Work out the finished part from the listing and answer in its coordinate system (mm). A direction names the side the tool comes from. Round coordinates to 2 decimals unless told otherwise and drop trailing zeros. Loops run counter-clockwise (first coordinate to the right, second up) from the corner with the lowest first, then second, coordinate; pieces in that order, holes last. Notation, with made-up numbers: (64, -17) - (108, -17) arc R16 ccw to (108, -13) - close; hole circle Ø5 at (81, -19). An arc over 180 degrees is marked (long way). Answer as CSV lines item,"result". Start each with the question number.
Q1. The mould has two halves that part along Z. Classify faces 4 (the face through (25, -2, -8.365)), 5 (the face through (37, -2, 12.675)), 6 (the face through (-6.727, 4.465, 32.917)), 7 (the face through (-9, 7, -5)): +Z half, -Z half, draft (parallel to the pull), parting line (faces both ways), or undercut.
Q2. Section B-B on y = 2.75 is taken. Write down the section's boundary in (x, z).
Q3. Section C-C on y = -1 is taken. Write down the section's boundary in (x, z).
Q4. Section A-A on x = 37 is taken. Write down the section's boundary in (y, z), then the cut area to 3 significant figures.
Q5. Each of these flat-tipped pins is pushed along its axis until it touches: pin 1 Ø1 at (y, z) = (3.5, -1.5) entering from -X; pin 2 Ø6 at (y, z) = (4.5, 0) entering from +X; pin 3 Ø3.5 at (x, z) = (-6.64, 34.92) entering from +Y. Where does it stop, or does it pass through?
Q6. Section D-D on z = 10.5 is taken. Write down the section's boundary in (x, y).
Q7. For faces 1 (the face through (15.52, -2.22, 15.33)), 2 (the face through (53.99, 4.46, 33.44)), 3 (the face through (24, -4.5, 16)), determine the directions among +Z, -Z, +X, -X, +Y, -Y from which every point of the face is accessible in a straight line to the end or side of a thin tool.
Q8. Straight lines are drawn through the part: L1, parallel to X at y = -2, z = 13.5; L2, parallel to Y at x = 21, z = 31; L3, parallel to X at y = -3.5, z = -4.5. For each, find the intervals that lie inside material, in ascending order. Write a range as [from, to].
Autodesk Inventor part; units mm, degrees
ref_plane "YZ Plane" through (0, 0, 0) normal (1, 0, 0) x (0, 1, 0)
ref_plane "XZ Plane" through (0, 0, 0) normal (0, 1, 0) x (-1, 0, 0)
ref_plane "XY Plane" through (0, 0, 0) normal (0, 0, 1) x (1, 0, 0)
sketch "proto-board hole layout" plane through (0, 0, 0) normal (0, 1, 0) x (-1, 0, 0)
  circle A0 centre (6.6395, -4.3647) radius 1.49
  circle A1 centre (-55.3405, -4.3647) radius 1.49
  circle A2 centre (-55.3405, 34.9153) radius 1.49
  circle A3 centre (6.6395, 34.9153) radius 1.49
  line L0 (5.1495, -4.3647) -> (-53.8505, -4.3647) construction
  line L1 (5.1495, 34.9153) -> (-53.8505, 34.9153) construction
  line L2 (-55.3405, 33.4253) -> (-55.3405, -2.8747) construction
  line L3 (6.6395, 33.4253) -> (6.6395, -2.8747) construction
  dimension "d0" = 2.98
  dimension "d1" = 59
  dimension "d2" = 36.3
sketch "Sketch3" plane through (0, 0, 0) normal (0, 1, 0) x (-1, 0, 0)
  circle A0 centre (6.6395, -4.3647) radius 1.49
  circle A1 centre (6.6395, -4.3647) radius 4
  point P0 (0, 0)
  dimension "d15" = 8
extrude "Extrusion2" add sketch "Sketch3" along normal blind 7 contours A0 | A1
sketch "Sketch4" plane through (-6.6395, 7, -4.3647) normal (0, 1, 0) x (1, 0, 0)
  circle A0 centre (0, 0) radius 4 construction
  point P0 (6.6395, -4.3647)
hole "Hole1" at (-6.6395, 7, -4.3647) direction (0, -1, 0) diameter 4 depth 5 tip angle 118
chamfer "Chamfer1" distance 1 distance2 2 1 edges at (-2.6395, 7, -4.3647) measured on face at (-9.9293, 7, -4.7642)
pattern_sketch "Sketch Driven Pattern1" from (-6.6395, 0, -4.3647) copies at (55.3405, 0, -4.3647) at (55.3405, 0, 34.9153) at (-6.6395, 0, 34.9153)
sketch "Sketch5" plane through (-6.6395, 0, 34.9153) normal (0, -1, 0) x (1, 0, 0)
  circle A0 centre (0, 0) radius 4
  circle A1 centre (61.98, 0) radius 4
  circle A2 centre (61.98, -39.28) radius 4
  circle A3 centre (0, -39.28) radius 4
  line L0 (-4, 4) -> (65.98, 4)
  line L1 (65.98, 4) -> (65.98, -43.28)
  line L2 (65.98, -43.28) -> (-4, -43.28)
  line L3 (-4, -43.28) -> (-4, 4)
  point P0 (6.6395, -34.9153)
  point P1 (-4, 0)
  point P2 (-4, -39.28)
  point P3 (0, -43.28)
  point P4 (61.98, -43.28)
  point P5 (65.98, -39.28)
  point P6 (65.98, 0)
  point P7 (61.98, 4)
  point P8 (0, 4)
extrude "Extrusion3" add sketch "Sketch5" along normal blind 4.5 contours A0 | A0 L0 A1 L1 A2 L2 A3 L3 | A1 | A3 | A2
sketch "Sketch6" plane through (-6.6395, 0, 34.9153) normal (0, 1, 0) x (1, 0, 0)
  line L0 (0, 43.28) -> (61.98, 43.28)
  line L1 (30.99, 43.28) -> (30.99, -4) construction
  line L2 (61.98, -4) -> (0, -4)
  line L3 (-4, 0) -> (-4, 39.28)
  line L4 (-4, 19.64) -> (65.98, 19.64) construction
  line L5 (65.98, 39.28) -> (65.98, 0)
  line L6 (19.56, 19.64) -> (17.02, 19.64) construction
  line L7 (19.56, 17.04) -> (17.02, 17.04)
  line L8 (17.02, 22.24) -> (19.56, 22.24)
  arc A0 (19.56, 17.04) -> (19.56, 22.24) centre (19.56, 19.64) ccw
  arc A1 (17.02, 22.24) -> (17.02, 17.04) centre (17.02, 19.64) ccw
  line L9 (42.42, 17.04) -> (44.96, 17.04)
  line L10 (44.96, 22.24) -> (42.42, 22.24)
  arc A2 (42.42, 22.24) -> (42.42, 17.04) centre (42.42, 19.64) ccw
  arc A3 (44.96, 17.04) -> (44.96, 22.24) centre (44.96, 19.64) ccw
  point P0 (6.6395, 34.9153)
  point P1 (18.29, 19.64)
  point P2 (18.29, 22.24)
  point P3 (18.29, 17.04)
  dimension "d21" = 11.43
  dimension "d22" = 13.97
  dimension "d23" = 5.2
extrude "Extrusion4" cut sketch "Sketch6" against normal blind 4.5
properties part number "proto-board_standoffs_plate_t-slot-2inx1in"
Findings:
1,face 4,"-Z half"
1,face 5,"undercut"
1,face 6,"undercut"
1,face 7,"draft"
2,outline,"circle Ø8 at (-6.64, -4.36); circle Ø8 at (-6.64, 34.92); circle Ø8 at (55.34, -4.36); circle Ø8 at (55.34, 34.92); hole circle Ø4 at (-6.64, -4.36); hole circle Ø4 at (-6.64, 34.92); hole circle Ø4 at (55.34, -4.36); hole circle Ø4 at (55.34, 34.92)"
3,outline,"(-10.64, -4.36) arc R4 ccw to (-6.64, -8.36) - (55.34, -8.36) arc R4 ccw to (59.34, -4.36) - (59.34, 34.92) arc R4 ccw to (55.34, 38.92) - (-6.64, 38.92) arc R4 ccw to (-10.64, 34.92) - close; hole (10.38, 12.68) - (12.92, 12.68) arc R2.6 ccw to (12.92, 17.88) - (10.38, 17.88) arc R2.6 ccw to start; hole (35.78, 12.68) - (38.32, 12.68) arc R2.6 ccw to (38.32, 17.88) - (35.78, 17.88) arc R2.6 ccw to start"
4,outline,"(-4.5, -8.36) - (0, -8.36) - (0, 12.68) - (-4.5, 12.68) - close; (-4.5, 17.88) - (0, 17.88) - (0, 38.92) - (-4.5, 38.92) - close"
4,area,"189 mm^2"
5,pin 1,"stops at x = -9.87"
5,pin 2,"stops at x = 59.1"
5,pin 3,"stops at y = 1.85"
6,outline,"(-10.64, -4.5) - (59.34, -4.5) - (59.34, 0) - (-10.64, 0) - close"
7,face 1,"+Y, -Y"
7,face 2,"+Y"
7,face 3,"+Z, -Z, +X, -X, -Y"
8,L1,"x = [-10.64, 8.48], [14.82, 33.88], [40.22, 59.34]"
8,L2,"y = [-4.5, 0]"
8,L3,"x = [-10.64, 59.34]"
